Build history of the part. All positions in model axes, mm. Face numbers are marked on the shaded views. Round coordinates to 2 decimals unless told otherwise and drop trailing zeros. Write each loop counter-clockwise with the first axis right and the second up, starting at its lowest first coordinate (ties: lowest second). Pieces come first, ordered by that corner, then holes. Notation, with made-up numbers: (-4.5, 82.25) -> (7.5, 82.25) arc R22 ccw to (7.5, 118.25) -> close; hole circle Ø4 at (67, -14). An arc over 180 degrees is marked (long way). Return JSON: item names as keys, results as strings.
Autodesk Inventor part; units mm, degrees
ref_plane "YZ Plane" through (0, 0, 0) normal (1, 0, 0) x (0, 1, 0)
ref_plane "XZ Plane" through (0, 0, 0) normal (0, 1, 0) x (-1, 0, 0)
ref_plane "XY Plane" through (0, 0, 0) normal (0, 0, 1) x (1, 0, 0)
sketch "Esboço1" plane through (0, 0, 0) normal (0, 0, 1) x (1, 0, 0)
  line L0 (1.0701, 11.9834) -> (-0.8299, 11.9834)
  line L1 (-64.2299, 11.9834) -> (-64.2299, -10.0166)
  line L2 (-64.2299, -10.0166) -> (5.7701, -10.0166)
  line L3 (5.7701, -10.0166) -> (5.7701, 11.9834)
  line L4 (-61.2299, -10.5466) -> (-61.2299, 13.5834)
  line L5 (2.7701, 57.5834) -> (2.7701, -6.4166)
  line L6 (-31.3299, 21.5834) -> (-37.5299, 21.5834)
  line L7 (5.7701, -10.0166) -> (2.8701, -10.0166)
  line L8 (-59.5299, 11.9834) -> (-57.6299, 11.9834)
  line L9 (-38.8299, 21.5834) -> (-38.8299, 12.0834)
  line L10 (-19.6299, 21.5834) -> (-19.6299, 12.0834)
  line L11 (-19.6299, 11.9834) -> (-19.6299, 21.5834)
  line L12 (-19.6299, 21.5834) -> (-38.8299, 21.5834)
  line L13 (-38.8299, 21.5834) -> (-38.8299, 11.9834)
  line L14 (-64.2299, 11.9834) -> (-38.8299, 11.9834)
  line L15 (-19.6299, 11.9834) -> (5.7701, 11.9834)
  point P0 (0, 0)
extrude "Extrusão1" add sketch "Esboço1" along normal blind 1.5
properties part number "pcb sensor de cor"
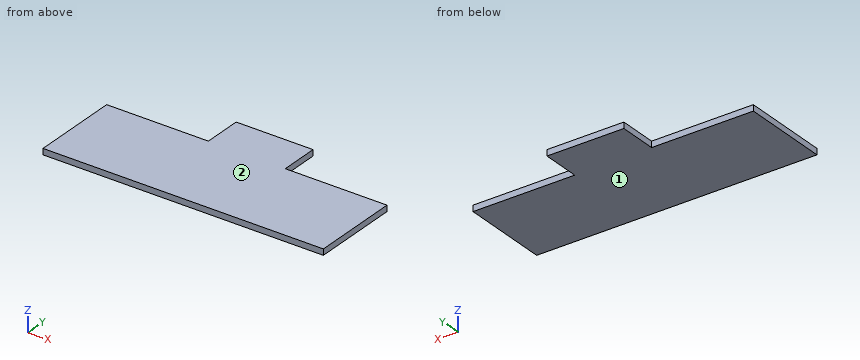
Q1. Wall check: L1, parallel to Y at x = -0.5, z = 0.5; L2, parallel to X at y = 20, z = 0.75. Give the ranges that are in metal, low to high.
Verdict:
{"L1": "y = -10.02 to 11.98", "L2": "x = -38.83 to -19.63"}
Q2. Pin check, flat tip, straight feed: pin 1 Ø0.8 at (x, z) = (-45.5, 0.5) entering from +Y. Stop position of the tip, or through.
Verdict:
{"pin 1": "stops at y = 11.98"}
Q3. Saw through at C-C on y = 13.5. List the corners of the cut face in (x, z), then the cut area to 3 significant figures.
Verdict:
{"outline": "(-38.83, 0) -> (-19.63, 0) -> (-19.63, 1.5) -> (-38.83, 1.5) -> close", "area": "28.8 mm²"}
Q4. Saw through at B-B on x = -2. List the corners of the cut face in (y, z), then the cut area to 3 significant figures.
Verdict:
{"outline": "(-10.02, 0) -> (11.98, 0) -> (11.98, 1.5) -> (-10.02, 1.5) -> close", "area": "33.0 mm²"}
Q5. Saw through at A-A on z = 0.8. List the corners of the cut face in (x, y), then the cut area to 3 significant figures.
Verdict:
{"outline": "(-64.23, -10.02) -> (5.77, -10.02) -> (5.77, 11.98) -> (-19.63, 11.98) -> (-19.63, 21.58) -> (-38.83, 21.58) -> (-38.83, 11.98) -> (-64.23, 11.98) -> close", "area": "1,720 mm²"}
Q6. Two-plate mould, pull along Z, no slides. Class the marked faces 1 and 2: +Z half, -Z half, draft (parallel to the pull), parting line (faces both ways), or undercut.
Verdict:
{"face 1": "-Z half", "face 2": "+Z half"}
